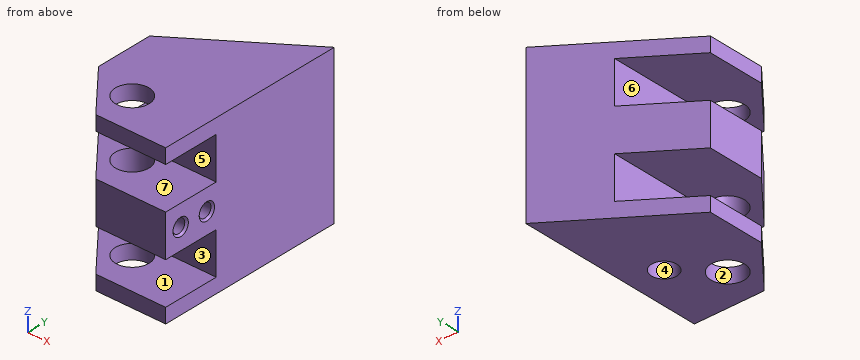
```python
from build123d import *

# Parameters (mm, degrees)
BOSS_EXTRUDE1_DEPTH             = 18.5
SKETCH2_R                       = 2
CUT_EXTRUDE1_DEPTH              = 19.5
SKETCH2_3_R                     = 1.5
CUT_EXTRUDE2_DEPTH              = 11
CUT_EXTRUDE3_DEPTH              = 19.5
CUT_EXTRUDE4_DEPTH              = 19.5
SKETCH7_W                       = 5
SKETCH7_H                       = 6.75
CUT_EXTRUDE5_DEPTH              = 14.5
M2X0_4_TAPPED_HOLE1_D           = 1.6
M2X0_4_TAPPED_HOLE1_DEPTH       = 5
M2X0_4_TAPPED_HOLE1_CSINK_D     = 2.05
M2X0_4_TAPPED_HOLE1_CSINK_ANGLE = 90
M2X0_4_TAPPED_HOLE1_TIP         = 0.480688495
SKETCH11_W                      = 7
SKETCH11_H                      = 5
CUT_EXTRUDE6_DEPTH              = 16.75


with BuildPart() as part:
    # Sketch1 → Boss-Extrude1 (new body)
    with BuildSketch(Plane.XY):
        Polygon((-7.276445285, -10.518598852), (2.223554715, -16.00342641), (6.223554715, -16.00342641), (6.223554715, 8.99657359), (-7.276445285, -0.518598852), align=None)
    extrude(amount=BOSS_EXTRUDE1_DEPTH)

    # Sketch2 → Cut-Extrude1 (cut, through all)
    with BuildSketch(Plane(origin=(0, 0, 0), x_dir=(-1, 0, 0), z_dir=(0, 0, -1))):
        with Locations((1.776445285, -9.00342641)):
            Circle(SKETCH2_R)
    extrude(amount=-CUT_EXTRUDE1_DEPTH, mode=Mode.SUBTRACT)

    # Sketch2<3> → Cut-Extrude2 (cut)
    with BuildSketch(Plane(origin=(0, 0, 0), x_dir=(-1, 0, 0), z_dir=(0, 0, -1))):
        with Locations((-2.223554715, -5.00342641)):
            Circle(SKETCH2_3_R)
    extrude(amount=-CUT_EXTRUDE2_DEPTH, mode=Mode.SUBTRACT)

    # Sketch5 → Cut-Extrude3 (cut, through all)
    with BuildSketch(Plane(origin=(0, 0, 0), x_dir=(-1, 0, 0), z_dir=(0, 0, -1))):
        Polygon((-6.223554715, -13.50342641), (2.106572304, -13.50342641), (-2.223554715, -16.00342641), (-6.223554715, -16.00342641), align=None)
    extrude(amount=-CUT_EXTRUDE3_DEPTH, mode=Mode.SUBTRACT)

    # Sketch6 → Cut-Extrude4 (cut, through all)
    with BuildSketch(Plane(origin=(0, 0, 0), x_dir=(-1, 0, 0), z_dir=(0, 0, -1))):
        Polygon((2.106572304, -13.50342641), (7.276445285, -7.342211711), (7.276445285, -10.518598852), align=None)
    extrude(amount=-CUT_EXTRUDE4_DEPTH, mode=Mode.SUBTRACT)

    # Sketch7 → Cut-Extrude5 (cut, through all)
    with BuildSketch(Plane(origin=(6.223554715, 0, 0), x_dir=(0, 0, -1), z_dir=(1, 0, 0))):
        with Locations((-14.25, -10.12842641)):
            Rectangle(SKETCH7_W, SKETCH7_H)
        with Locations((-4.25, -10.12842641)):
            Rectangle(SKETCH7_W, SKETCH7_H)
    extrude(amount=-CUT_EXTRUDE5_DEPTH, mode=Mode.SUBTRACT)

    # M2x0.4 Tapped Hole1
    with Locations(Plane(origin=(6.223554715, 0, 0), x_dir=(0, 0, -1), z_dir=(1, 0, 0))):
        with Locations((-9.25, -8.00342641), (-9.25, -11.50342641)):
            CounterSinkHole(M2X0_4_TAPPED_HOLE1_D / 2, M2X0_4_TAPPED_HOLE1_CSINK_D / 2, depth=M2X0_4_TAPPED_HOLE1_DEPTH, counter_sink_angle=M2X0_4_TAPPED_HOLE1_CSINK_ANGLE)
            with Locations((0, 0, -(M2X0_4_TAPPED_HOLE1_DEPTH + M2X0_4_TAPPED_HOLE1_TIP / 2))):  # 118° drill point
                Cone(0, M2X0_4_TAPPED_HOLE1_D / 2, M2X0_4_TAPPED_HOLE1_TIP, mode=Mode.SUBTRACT)

    # Sketch11 → Cut-Extrude6 (cut, through all)
    with BuildSketch(Plane.XZ.offset(6.75342641)):
        with Locations((-3.776445285, 14.25)):
            Rectangle(SKETCH11_W, SKETCH11_H)
        with Locations((-3.776445285, 4.25)):
            Rectangle(SKETCH11_W, SKETCH11_H)
    extrude(amount=-CUT_EXTRUDE6_DEPTH, mode=Mode.SUBTRACT)


solid = part.part
```
Source: CAD feature listing. Evaluate the final solid. Frame: model axes, mm. Face numbers are marked on the shaded views. A direction names the side the tool comes from. Coordinates: 2 decimals unless noted, no trailing zeros. Write each loop counter-clockwise with the first axis right and the second up, starting at its lowest first coordinate (ties: lowest second). Pieces come first, ordered by that corner, then holes. Notation, with made-up numbers: M -37,-2 L -6,-2 A21 cw -6,30 Z; hole C -37.75,46.25 d4. An arc over 180 degrees is marked long. Answer as a JSON object with one key per item and string values.
1. Contact query for flat-ended pins moving along their axis: P1, Ø1.4, axis at y = -11.5, z = 9.25, coming from the -X side (3 decimals); P2, Ø2.5, axis at x = -1.78, y = -9, coming from the +Z side; P3, Ø2.5, axis at y = 0, z = 13.5, coming from the -X side; P4, Ø2.5, axis at x = 3.5, z = 13.5, coming from the -Y side. Output: stop coordinate, or through.
Evaluation:
{"P1": "x = -4.375", "P2": "through", "P3": "x = -0.28", "P4": "y = -6.75"}
2. Draft query along Y for the marked faces 1, 2 and 3. Return one class per face: released by +Y, released by -Y, zero draft, split by the parting line, or undercut.
Evaluation:
{"face 1": "zero draft", "face 2": "undercut", "face 3": "released by -Y"}
3. Access query for the marked faces 4, 5, 6 and 7. Directions: +Z, -Z, +X, -X, +Y, -Y. A direction counts if a zero-diameter tool reaches every point of the face in a straight line with its end or side. Return the directions, or none.
Evaluation:
{"face 4": "-Z", "face 5": "+X, -X, -Y", "face 6": "-X, +Y, -Y", "face 7": "-X, -Y"}
4. Ray query, L1, parallel to Z at x = -0.5, y = 2; L2, parallel to Z at x = 5, y = -8.5; L3, parallel to Y at x = 3.45, z = 9.25. Return the intervals inside material, ascending.
Evaluation:
{"L1": "0 to 1.75, 6.75 to 11.75, 16.75 to 18.5", "L2": "0 to 1.75, 6.75 to 8.62, 9.88 to 11.75, 16.75 to 18.5", "L3": "-13.5 to -12.3, -10.7 to -8.8, -7.2 to -5.87, -4.14 to 7.04"}
5. Cut plane A-A on y = -10. Output: boundary loops of the cut face in (x, z).
Evaluation:
{"outline": "M -5.05,0 L -3.51,0 L -3.51,1.75 L -5.05,1.75 Z; M -5.05,6.75 L -3.51,6.75 L -3.51,11.75 L -5.05,11.75 Z; M -5.05,16.75 L -3.51,16.75 L -3.51,18.5 L -5.05,18.5 Z; M -0.04,0 L 6.22,0 L 6.22,1.75 L -0.04,1.75 Z; M -0.04,6.75 L 6.22,6.75 L 6.22,11.75 L -0.04,11.75 Z; M -0.04,16.75 L 6.22,16.75 L 6.22,18.5 L -0.04,18.5 Z"}
6. Cut plane D-D on y = 0.5. Output: boundary loops of the cut face in (x, z).
Evaluation:
{"outline": "M -5.83,0 L 6.22,0 L 6.22,18.5 L -5.83,18.5 L -5.83,16.75 L -0.28,16.75 L -0.28,11.75 L -5.83,11.75 L -5.83,6.75 L -0.28,6.75 L -0.28,1.75 L -5.83,1.75 Z"}
7. Cut plane B-B on x = 2.25. Output: boundary loops of the cut face in (y, z), plus the area to 3 significant figures.
Evaluation:
{"outline": "M -13.5,0 L -6.5,0 L -6.5,11 L -3.5,11 L -3.5,0 L 6.2,0 L 6.2,18.5 L -13.5,18.5 L -13.5,16.75 L -6.75,16.75 L -6.75,11.75 L -13.5,11.75 L -13.5,6.75 L -6.75,6.75 L -6.75,1.75 L -13.5,1.75 Z; hole C -11.5,9.25 d1.6; hole C -8,9.25 d1.6", "area": "260 mm^2"}
8. Cut plane C-C on z = 7.75. Output: boundary loops of the cut face in (x, y), plus the area to 3 significant figures.
Evaluation:
{"outline": "M -7.28,-7.34 L -2.11,-13.5 L 6.22,-13.5 L 6.22,9 L -7.28,-0.52 Z; hole C -1.78,-9 d4; hole C 2.22,-5 d3", "area": "204 mm^2"}
